Design review of the part built by this model. Coordinates are the model's own, in mm. A direction names the side the tool comes from. Give positions to 0.01 mm unless a question says otherwise; leave off trailing zeros. Write each loop counter-clockwise with the first axis right and the second up, starting at its lowest first coordinate (ties: lowest second). Pieces come first, ordered by that corner, then holes. Notation, with made-up numbers: (54.5, 0) -> (96.5, 0) arc R13 cw to (96.5, 16) -> close; hole circle Ø9 at (57.5, 85). An arc over 180 degrees is marked (long way). Put each result on its own line as item: value. Start each with the question number.
from build123d import *

# Parameters (mm, degrees)
SKETCH1_W                      = 152.4
SKETCH1_H                      = 19.05
BASE_FLANGE1_DEPTH             = 3.175
EDGE_FLANGE1_STRIP_W           = 19.05
EDGE_FLANGE1_STRIP_H           = 3.175
EDGE_FLANGE1_STRIP_CUT_DEPTH   = 152.4
EDGE_FLANGE1_STRIP_2_W         = 19.05
EDGE_FLANGE1_STRIP_2_H         = 3.175
EDGE_FLANGE1_STRIP_CUT_2_DEPTH = 152.4
EDGE_FLANGE1_DEPTH             = 152.4
EDGE_FLANGE1_BEND_DEPTH        = 152.4
CUT_EXTRUDE1_DEPTH             = 87.08071453
F_30_0_1285_DIAMETER_HOLE1_D   = 3.2639


# Sheet-metal steps are written as plain solids
with BuildPart() as part:
    # Sketch1 → Base-Flange1 (new body)
    with BuildSketch(Plane(origin=(0, 0, 0), x_dir=(1, 0, 0), z_dir=(0, 1, 0))):
        Rectangle(SKETCH1_W, SKETCH1_H)
    extrude(amount=-BASE_FLANGE1_DEPTH)

    # Edge-Flange1 strip (across the edge) → Edge-Flange1 strip cut (cut)
    with BuildSketch(Plane(origin=(-76.2, 0, 9.525), x_dir=(0, 0, -1), z_dir=(1, 0, 0))):
        with Locations((-6.35, -1.5875)):
            Rectangle(EDGE_FLANGE1_STRIP_W, EDGE_FLANGE1_STRIP_H)
    extrude(amount=EDGE_FLANGE1_STRIP_CUT_DEPTH, mode=Mode.SUBTRACT)

    # Edge-Flange1 strip 2 (across the edge) → Edge-Flange1 strip cut 2 (cut)
    with BuildSketch(Plane(origin=(76.2, 0, -9.525), x_dir=(0, 0, 1), z_dir=(-1, 0, 0))):
        with Locations((-6.35, -1.5875)):
            Rectangle(EDGE_FLANGE1_STRIP_2_W, EDGE_FLANGE1_STRIP_2_H)
    extrude(amount=EDGE_FLANGE1_STRIP_CUT_2_DEPTH, mode=Mode.SUBTRACT)

    # Edge-Flange1 section (across the edge) → Edge-Flange1 (add)
    with BuildSketch(Plane(origin=(-76.2, 0, 9.525), x_dir=(0, 0, -1), z_dir=(1, 0, 0))):
        with BuildLine():
            Line((-3.175, 3.175), (-3.175, 30.95625))
            Line((-3.175, 30.95625), (0, 30.95625))
            Line((0, 30.95625), (0, 3.175))
            ThreePointArc((0, 3.175), (0.92993597, 0.92993597), (3.175, 0))
            Line((3.175, 0), (3.175, -3.175))
            ThreePointArc((3.175, -3.175), (-1.315128061, -1.315128061), (-3.175, 3.175))
        make_face()
    extrude(amount=EDGE_FLANGE1_DEPTH)

    # Edge-Flange1 section 2 (across the edge) → Edge-Flange1 bend (add)
    with BuildSketch(Plane(origin=(76.2, 0, -9.525), x_dir=(0, 0, 1), z_dir=(-1, 0, 0))):
        with BuildLine():
            Line((-3.175, 3.175), (-3.175, 30.95625))
            Line((-3.175, 30.95625), (0, 30.95625))
            Line((0, 30.95625), (0, 3.175))
            ThreePointArc((0, 3.175), (0.92993597, 0.92993597), (3.175, 0))
            Line((3.175, 0), (3.175, -3.175))
            ThreePointArc((3.175, -3.175), (-1.315128061, -1.315128061), (-3.175, 3.175))
        make_face()
    extrude(amount=EDGE_FLANGE1_BEND_DEPTH)

    # Sketch12 → Cut-Extrude1 (cut, through all)
    with BuildSketch(Plane(origin=(0, 0, -12.7), x_dir=(-1, 0, 0), z_dir=(0, 0, -1))):
        Polygon((76.2, 30.95625), (0, 30.95625), (76.2, 22.935197368), align=None)
        Polygon((-76.2, 22.935197368), (0, 30.95625), (-76.2, 30.95625), align=None)
    extrude(amount=-CUT_EXTRUDE1_DEPTH, mode=Mode.SUBTRACT)

    # #30 (0.1285) Diameter Hole1 (through all)
    with Locations(Plane(origin=(0, 0, -12.7), x_dir=(-1, 0, 0), z_dir=(0, 0, -1))):
        with Locations((-69.498892921, 14.062952351), (-56.868673669, 15.392449114), (-44.238454417, 16.721945878), (-31.608235165, 18.051442641), (-18.978015912, 19.380939405), (-6.34779666, 20.710436168), (6.34779666, 20.710436168), (18.978015912, 19.380939405), (31.608235165, 18.051442641), (44.238454417, 16.721945878), (56.868673669, 15.392449114), (69.498892921, 14.062952351)):
            Hole(F_30_0_1285_DIAMETER_HOLE1_D / 2)


solid = part.part
Q1. Take a section at D-D on y = 26. Give the boundary of the cut face in (x, z) (3 decimals).
Q2. To check wall thickness, follow probe 1 along Z at (x, y) = (-11.5, 28) (3 decimals); probe 2 along Y at (x, z) = (-1, -4) (3 decimals); probe 3 along Y at (x, z) = (-35, -8.5). State the ranges of each line that lie inside material, in increasing order. Write a range as from..to.
Q3. Take a section at C-C on z = -2.75. Give the boundary of the cut face in (x, y) (3 decimals).
Q4. Take a section at B-B on x = 57. Give the boundary of the cut face in (y, z) (3 decimals), then the cut area to 3 significant figures.
Q5. Take a section at A-A on y = 5. Give the boundary of the cut face in (x, z) (3 decimals).
Q6. Machinability: for faces 4 (the face through (-58.5, 15.46, -11.09)), 5 (the face through (-1, 0, 0)), which of the approach directions +Z, -Z, +X, -X, +Y, -Y give a long, thin tool a straight path to every point of the face, cutting with its end or side? Answer none if there is none.
Q7. Mouldability with a two-part tool opening along Y and no side actions: class faces 1 (the face through (31.4, 19.67, 11.13)), 2 (the face through (-1, -3.175, 0)), 3 (the face through (1, 14, -9.525)) as +Y half, -Y half, draft (parallel to the pull), parting line (faces both ways), or undercut.
Q8. For pin 1 (2 mm diameter, centred on x = 48.5, z = -9, fed in from +Y); pin 2 (4 mm diameter, centred on x = 11.5, z = -2, fed in from +Y), all flat-tipped, find the tip position at first contact; note any pin that passes through.
Result:
1. outline: (-47.084, -12.7) -> (47.084, -12.7) -> (47.084, -9.525) -> (-47.084, -9.525) -> close; (-47.084, 9.525) -> (47.084, 9.525) -> (47.084, 12.7) -> (-47.084, 12.7) -> close
2. probe 1: z = -12.7..-9.525, 9.525..12.7
2. probe 2: y = -3.175..0
2. probe 3: y = -2.8..0.84
3. outline: (-76.2, -3.175) -> (76.2, -3.175) -> (76.2, 0) -> (-76.2, 0) -> close
4. outline: (-3.175, -6.35) arc R6.35 ccw to (3.175, -12.7) -> (13.766, -12.7) -> (13.766, -9.525) -> (3.175, -9.525) arc R3.175 cw to (0, -6.35) -> (0, 6.35) arc R3.175 cw to (3.175, 9.525) -> (13.766, 9.525) -> (13.766, 12.7) -> (3.175, 12.7) arc R6.35 ccw to (-3.175, 6.35) -> close; (17.019, -12.7) -> (24.956, -12.7) -> (24.956, -9.525) -> (17.019, -9.525) -> close; (17.019, 9.525) -> (24.956, 9.525) -> (24.956, 12.7) -> (17.019, 12.7) -> close
4. area: 205 mm^2
5. outline: (-76.2, -12.7) -> (76.2, -12.7) -> (76.2, -9.525) -> (-76.2, -9.525) -> close; (-76.2, 9.525) -> (76.2, 9.525) -> (76.2, 12.7) -> (-76.2, 12.7) -> close
6. face 4: +Z, -Z
6. face 5: +X, -X, +Y
7. face 1: undercut
7. face 2: -Y half
7. face 3: draft
8. pin 1: stops at y = 25.94
8. pin 2: stops at y = 0
